Can you work these out from the model? Positions are in its coordinate system, mm. Face numbers are marked on the shaded views. A direction names the side the tool comes from. Give positions to 0.01 mm unless a question says otherwise; leave off trailing zeros. Write each loop counter-clockwise with the first axis right and the second up, starting at its lowest first coordinate (ties: lowest second). Pieces come first, ordered by that corner, then holes. Notation, with made-up numbers: M 80.25,-9.75 L 139.25,-9.75 A36 ccw 139.25,25.25 Z; hole C 16,64.5 d3. An arc over 180 degrees is marked long. Write each question's results on one line, items separated by ' | '.
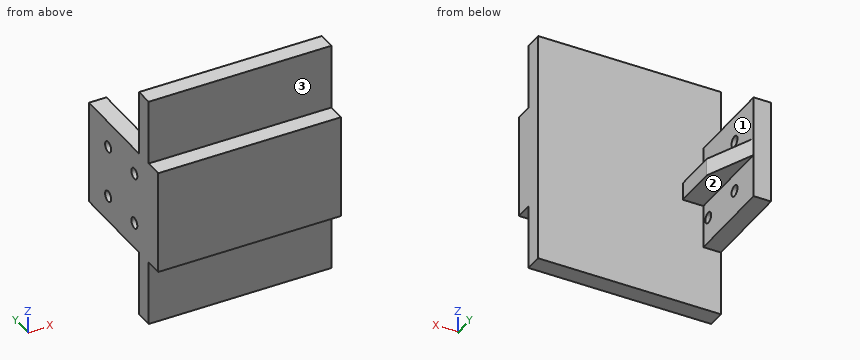
from build123d import *

# Parameters (mm, degrees)
EXTRUDE_1_DEPTH      = 24
SKETCH_2_W           = 42
SKETCH_2_H           = 4
EXTRUDE_2_DEPTH      = 15
EXTRUDE_3_DEPTH      = 2
EXTRUDE_3_DEPTH_BACK = 2
SKETCH_5_R           = 1.25
CUT_EXTRUDE_1_DEPTH  = 62.692787261


with BuildPart() as part:
    # Эскиз1 → Бобышка-Вытянуть1 (new body)
    with BuildSketch(Plane.XY):
        Polygon((0, 0), (0, 29), (4, 29), (4, 8), (42, 8), (42, 0), align=None)
    extrude(amount=-EXTRUDE_1_DEPTH)

    # Эскиз2 → Бобышка-Вытянуть2 (add)
    with BuildSketch(Plane.XY):
        with Locations((21, 6)):
            Rectangle(SKETCH_2_W, SKETCH_2_H)
    extrude_2 = extrude(amount=EXTRUDE_2_DEPTH)

    # Зеркальное отражение1: Бобышка-Вытянуть2 across plane
    add(extrude_2.mirror(Plane.XY.offset(-12)))

    # Эскиз4 → Бобышка-Вытянуть3 (add, two sides: drawn at the far end of the back side and taken through both)
    with BuildSketch(Plane(origin=(0, 0, -12), x_dir=(0, -1, 0), z_dir=(0, 0, 1)).offset(-EXTRUDE_3_DEPTH_BACK)):
        Polygon((-8, 8.75), (-18, 8.75), (-29, 4), (-8, 4), align=None)
    extrude(amount=EXTRUDE_3_DEPTH + EXTRUDE_3_DEPTH_BACK)

    # Эскиз5 → Вырез-Вытянуть1 (cut, through all)
    with BuildSketch(Plane(origin=(4, 0, 0), x_dir=(0, 0, -1), z_dir=(1, 0, 0))):
        with Locations(Location((6, 21, 0), (0, 0, 90))):
            Circle(SKETCH_5_R)
        with Locations(Location((6, 10, 0), (0, 0, 90))):
            Circle(SKETCH_5_R)
        with Locations(Location((18, 10, 0), (0, 0, 90))):
            Circle(SKETCH_5_R)
        with Locations(Location((18, 21, 0), (0, 0, 90))):
            Circle(SKETCH_5_R)
    extrude(amount=-CUT_EXTRUDE_1_DEPTH, mode=Mode.SUBTRACT)


solid = part.part
Item 1: I want a section at D-D, the plane y = 12.5. Please give me the cut outline in (x, z).
Geometry says:
outline: M 0,-24 L 4,-24 L 4,-14 L 8.75,-14 L 8.75,-10 L 4,-10 L 4,0 L 0,0 Z
Item 2: I want a section at C-C, the plane y = 21. Please give me the cut outline in (x, z).
Geometry says:
outline: M 0,-24 L 4,-24 L 4,-19.25 L 0,-19.25 Z; M 0,-16.75 L 4,-16.75 L 4,-14 L 7.45,-14 L 7.45,-10 L 4,-10 L 4,-7.25 L 0,-7.25 Z; M 0,-4.75 L 4,-4.75 L 4,0 L 0,0 Z
Item 3: I want a section at B-B, the plane x = 39. Please give me the cut outline in (y, z), and give its area (3 significant figures).
Geometry says:
outline: M 0,-24 L 4,-24 L 4,-39 L 8,-39 L 8,15 L 4,15 L 4,0 L 0,0 Z | area: 312 mm2
Item 4: If I drill on line 1 (Z direction, x = 1.7, y = 10); line 2 (Y direction, x = 21.5, z = -14); line 3 (X direction, y = 14.75, z = -4.5), over which ranges is the centre line in solid material (lowest first)? Write a range as from..to.
Geometry says:
line 1: z = -24..-19.25, -16.75..-7.25, -4.75..0 | line 2: y = 0..8 | line 3: x = 0..4
Item 5: For the marked faces 1, 2 and 3, which set-ups out of +Z, -Z, +X, -X, +Y, -Y let a thin tool reach every point of the face, with its end or its side?
Geometry says:
face 1: +Z, +X, +Y | face 2: -Z, +X, +Y | face 3: +Z, +X, -X, -Y
Item 6: I'm going to push flat-ended pins straight in: pin 1 (3 mm diameter, centred on x = 1, y = 15, fed in from -Z); pin 2 (1.2 mm diameter, centred on x = 21, y = 2, fed in from +Z); pin 3 (4.5 mm diameter, centred on x = 25.5, y = 2, fed in from -Z); pin 4 (2 mm diameter, centred on x = 32, z = -30.5, fed in from -Y). Where does each tip first touch, or does it pass through?
Geometry says:
pin 1: stops at z = -24 | pin 2: stops at z = 0 | pin 3: stops at z = -39 | pin 4: stops at y = 4
Item 7: I want a section at A-A, the plane z = -18. Please give me the cut outline in (x, y), and give its area (3 significant figures).
Geometry says:
outline: M 0,0 L 42,0 L 42,8 L 4,8 L 4,8.75 L 0,8.75 Z; M 0,11.25 L 4,11.25 L 4,19.75 L 0,19.75 Z; M 0,22.25 L 4,22.25 L 4,29 L 0,29 Z | area: 400 mm2
